Source: CAD feature listing. Evaluate the final solid. Frame: model axes, mm. Give positions to 0.01 mm unless a question says otherwise; leave off trailing zeros. Write each loop counter-clockwise with the first axis right and the second up, starting at its lowest first coordinate (ties: lowest second). Pieces come first, ordered by that corner, then holes. Notation, with made-up numbers: (28, -34) - (59, -34) arc R22 cw to (59, -16) - close; hole circle Ø9 at (-3.5, 15.25). An arc over 180 degrees is marked (long way). One line per question, with ' | ' between items. Start each with the question number.
(1) Section C-C, the plane y = 40. Return loops of the section in (x, z), plus the area to 3 significant figures.
(2) Pin query (flat end, axial travel): pin 1 (2.5 mm diameter, centred on x = 57, z = 3.5, fed in from -Y); pin 2 (4.5 mm diameter, centred on x = 15, y = 10, fed in from -Z); pin 3 (1.5 mm diameter, centred on y = 69.5, z = 2.5, fed in from +X). Return the tip coordinate at first contact, or that it passes through.
(3) Section B-B, the plane x = 62. Return loops of the section in (y, z).
(4) Section D-D, the plane y = 21.5. Return loops of the section in (x, z).
(5) Ray query, line 1 (Y direction, x = 15, z = 2.6); line 2 (Y direction, x = 16.5, z = 0.65); line 3 (X direction, y = 72.5, z = 3.95). Return the intervals inside material, ascending. Write a range as [from, to].
(6) Section A-A, the plane z = 1.05. Return loops of the section in (x, y), plus the area to 3 significant figures.
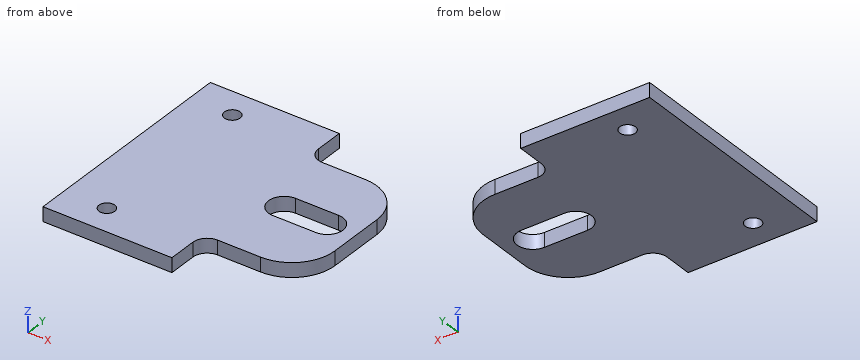
```python
from build123d import *

# Parameters (mm, degrees)
ESQUISSE1_R        = 2.75
BOSS_EXTRU_1_DEPTH = 5
CONG_1_R           = 5
CONG_2_R           = 15


with BuildPart() as part:
    # Esquisse1 → Boss.-Extru.1 (new body)
    with BuildSketch(Plane.XY):
        Polygon((0, 80), (0, 0), (45, 0), (45, 15), (80, 15), (80, 65), (45, 65), (45, 80), align=None)
        with Locations((15, 10)):
            Circle(ESQUISSE1_R, mode=Mode.SUBTRACT)
        with Locations((15, 70)):
            Circle(ESQUISSE1_R, mode=Mode.SUBTRACT)
        with BuildLine():
            ThreePointArc((70, 45.5), (75.5, 40), (70, 34.5))
            Line((70, 34.5), (55, 34.5))
            ThreePointArc((55, 34.5), (49.5, 40), (55, 45.5))
            Line((55, 45.5), (70, 45.5))
        make_face(mode=Mode.SUBTRACT)
    extrude(amount=BOSS_EXTRU_1_DEPTH)

    # Congé1
    cong_1_edges = [part.edges().sort_by_distance(p)[0] for p in [
        (45, 65, 2.5),
        (45, 15, 2.5),
    ]]
    fillet(cong_1_edges, radius=CONG_1_R)

    # Congé2
    cong_2_edges = [part.edges().sort_by_distance(p)[0] for p in [
        (80, 65, 2.5),
        (80, 15, 2.5),
    ]]
    fillet(cong_2_edges, radius=CONG_2_R)


solid = part.part
```
Check sheet entries:
1) outline: (0, 0) - (49.5, 0) - (49.5, 5) - (0, 5) - close; (75.5, 0) - (80, 0) - (80, 5) - (75.5, 5) - close | area: 270 mm²
2) pin 1: y = 15 | pin 2: through | pin 3: x = 45.16
3) outline: (15, 0) - (34.5, 0) - (34.5, 5) - (15, 5) - close; (45.5, 0) - (65, 0) - (65, 5) - (45.5, 5) - close
4) outline: (0, 0) - (77.36, 0) - (77.36, 5) - (0, 5) - close
5) line 1: [0, 7.25], [12.75, 67.25], [72.75, 80] | line 2: [0, 7.7], [12.3, 67.7], [72.3, 80] | line 3: [0, 13.85], [16.15, 45]
6) outline: (0, 0) - (45, 0) - (45, 10) arc R5 cw to (50, 15) - (65, 15) arc R15 ccw to (80, 30) - (80, 50) arc R15 ccw to (65, 65) - (50, 65) arc R5 cw to (45, 70) - (45, 80) - (0, 80) - close; hole circle Ø5.5 at (15, 10); hole circle Ø5.5 at (15, 70); hole (55, 34.5) - (70, 34.5) arc R5.5 ccw to (70, 45.5) - (55, 45.5) arc R5.5 ccw to start | area: 4,960 mm²
